```python
from build123d import *

# Parameters (mm, degrees)
SKETCH1_R           = 2.25
SKETCH1_R_2         = 15
BOSS_EXTRUDE1_DEPTH = 3


with BuildPart() as part:
    # Sketch1 → Boss-Extrude1 (new body)
    with BuildSketch(Plane(origin=(0, 0, 0), x_dir=(1, 0, 0), z_dir=(0, 1, 0))):
        Polygon((19, 21), (21, 19), (21, -19), (19, -21), (-19, -21), (-21, -19), (-21, 19), (-19, 21), align=None)
        with Locations((-16.263455967, 16.263455967)):
            Circle(SKETCH1_R, mode=Mode.SUBTRACT)
        with Locations((16.263455967, 16.263455967)):
            Circle(SKETCH1_R, mode=Mode.SUBTRACT)
        with Locations((16.263455967, -16.263455967)):
            Circle(SKETCH1_R, mode=Mode.SUBTRACT)
        with Locations((-16.263455967, -16.263455967)):
            Circle(SKETCH1_R, mode=Mode.SUBTRACT)
        Circle(SKETCH1_R_2, mode=Mode.SUBTRACT)
    extrude(amount=BOSS_EXTRUDE1_DEPTH)


solid = part.part
```
CAD build for the part. Positions are in the model's coordinates, mm. Give positions to 0.01 mm unless a question says otherwise; leave off trailing zeros. Order: outer loops, then holes, each group sorted by start corner. A loop starts at its lowest first (then second) coordinate and runs counter-clockwise, first axis right, second up. Notation, with made-up numbers: M -7.75,43 L 26.25,43 A27 ccw 26.25,69 Z; hole C -12.5,47 d4. An arc over 180 degrees is marked long. Put each result on its own line as item: value. Start each with the question number.
(1) Saw through at B-B, the plane z = -10. Write the cut outline in (x, y), then the cut area to 3 significant figures.
(2) Mould opens along X. For faces 1 (the cylindrical face through (-18.51, 1.48, 16.16)), 2 (the flat face through (10, 0, -14)), 3 (the flat face through (-20, 1, -20)) say: +X half, -X half, draft (parallel to the pull), parting line (faces both ways), or undercut.
(3) Drill centre lines: line 1 along X through (y, z) = (1.9, 0); line 2 along Z through (x, y) = (-16, 2.25); line 3 along Z through (x, y) = (1, 1.8). Where is each one in solid material? Low to high.
(4) Saw through at A-A, the plane x = 0. Write the cut outline in (y, z).
(5) Saw through at D-D, the plane x = -17. Write the cut outline in (y, z).
(6) Saw through at C-C, the plane y = 0.45. Write the cut outline in (x, z), then the cut area to 3 significant figures.
Check result:
1. outline: M -21,0 L -11.18,0 L -11.18,3 L -21,3 Z; M 11.18,0 L 21,0 L 21,3 L 11.18,3 Z
1. area: 58.9 mm2
2. face 1: undercut
2. face 2: draft
2. face 3: -X half
3. line 1: x = -21 to -15, 15 to 21
3. line 2: z = -21 to -18.5, -14.03 to 14.03, 18.5 to 21
3. line 3: z = -21 to -14.97, 14.97 to 21
4. outline: M 0,-21 L 3,-21 L 3,-15 L 0,-15 Z; M 0,15 L 3,15 L 3,21 L 0,21 Z
5. outline: M 0,-21 L 3,-21 L 3,-18.39 L 0,-18.39 Z; M 0,-14.14 L 3,-14.14 L 3,14.14 L 0,14.14 Z; M 0,18.39 L 3,18.39 L 3,21 L 0,21 Z
6. outline: M -21,-19 L -19,-21 L 19,-21 L 21,-19 L 21,19 L 19,21 L -19,21 L -21,19 Z; hole C -16.26,-16.26 d4.5; hole C -16.26,16.26 d4.5; hole C 0,0 d30; hole C 16.26,-16.26 d4.5; hole C 16.26,16.26 d4.5
6. area: 986 mm2
